from build123d import *

# Parameters (mm, degrees)
F1_DEPTH = 50
F4_DEPTH = 31
F5_R     = 26
F6_DEPTH = 15


with BuildPart() as f1:
    # F0 (on Front) → F1 (new body)
    with BuildSketch(Plane.XZ):
        with BuildLine():
            ThreePointArc((55.5, 51.9206124771), (30.2492433933, 69.7207521053), (0, 76))
            ThreePointArc((0, 76), (-76, 0), (0, -76))
            ThreePointArc((0, -76), (30.2492433933, -69.7207521053), (55.5, -51.9206124771))
            ThreePointArc((55.5, -51.9206124771), (35, 0), (55.5, 51.9206124771))
        make_face()
        with BuildLine():
            ThreePointArc((111, 76), (80.7507566067, 69.7207521053), (55.5, 51.9206124771))
            ThreePointArc((55.5, 51.9206124771), (70.6894617323, 27.9105714739), (76, 0))
            ThreePointArc((76, 0), (70.6894617323, -27.9105714739), (55.5, -51.9206124771))
            ThreePointArc((55.5, -51.9206124771), (80.7507566067, -69.7207521053), (111, -76))
            ThreePointArc((111, -76), (164.7401153702, -53.7401153702), (187, 0))
            ThreePointArc((187, 0), (164.7401153702, 53.7401153702), (111, 76))
        make_face()
        with BuildLine():
            ThreePointArc((76, 0), (70.6894617323, 27.9105714739), (55.5, 51.9206124771))
            ThreePointArc((55.5, 51.9206124771), (35, 0), (55.5, -51.9206124771))
            ThreePointArc((55.5, -51.9206124771), (70.6894617323, -27.9105714739), (76, 0))
        make_face()
        with BuildLine():
            Line((111, 76), (0, 76))
            ThreePointArc((0, 76), (30.2492433933, 69.7207521053), (55.5, 51.9206124771))
            ThreePointArc((55.5, 51.9206124771), (80.7507566067, 69.7207521053), (111, 76))
        make_face()
        with BuildLine():
            ThreePointArc((55.5, -51.9206124771), (30.2492433933, -69.7207521053), (0, -76))
            Line((0, -76), (111, -76))
            ThreePointArc((111, -76), (80.7507566067, -69.7207521053), (55.5, -51.9206124771))
        make_face()
    extrude(amount=F1_DEPTH)

    # F3 (on offset) → F4 (cut)
    with BuildSketch(Plane.XZ.offset(19)):
        with BuildLine():
            Line((111, 64), (0, 64))
            ThreePointArc((0, 64), (-64, 0), (0, -64))
            Line((0, -64), (111, -64))
            ThreePointArc((111, -64), (175, 0), (111, 64))
        make_face()
    extrude(amount=F4_DEPTH, mode=Mode.SUBTRACT)

    # F5 (on face) → F6 (cut)
    with BuildSketch(Plane.XZ.offset(19)):
        Circle(F5_R)
    extrude(amount=-F6_DEPTH, mode=Mode.SUBTRACT)

    # F8 (on offset) → F9 (revolve, cut)
    with BuildSketch(Plane.YZ.offset(111)):
        Polygon((-19, 0), (0, 0), (0, 11), (-2, 11), (-2, 18.5), (-7, 18.5), (-7, 23.5), (-19, 23.5), align=None)
    revolve(axis=Axis((111, -31.2652774155, 0), (0, -1, 0)), mode=Mode.SUBTRACT)


solid = f1.part
For this review, take the finished solid that the model builds, in its own axes (mm). A direction names the side the tool comes from. Coordinates: 2 decimals unless noted, no trailing zeros. Loops run counter-clockwise (first coordinate to the right, second up) from the corner with the lowest first, then second, coordinate; pieces in that order, holes last. Notation, with made-up numbers: (-7.5, 80) -> (30.5, 80) arc R19 cw to (30.5, 89) -> close; hole circle Ø5 at (16, 56.5). An arc over 180 degrees is marked (long way). Write each question's results on one line, items separated by ' | '.
Q1. To check wall thickness, follow line 1 along Z through (x, y) = (5, -46.5); line 2 along X through (y, z) = (-40.5, -2.5); line 3 along X through (y, z) = (-8, 3). State the ranges of each line that lie inside material, in increasing order. Write a range as [from, to].
Taken from the geometry:
line 1: [-76, -64], [64, 76] | line 2: [-75.96, -63.95], [174.95, 186.96] | line 3: [-75.94, -25.83], [25.83, 87.69], [134.31, 186.94]
Q2. Add section B-B, the plane x = 46.5. State the section outline as (y, z) points, then the cut area to 3 significant figures.
Taken from the geometry:
outline: (-50, -76) -> (0, -76) -> (0, 76) -> (-50, 76) -> (-50, 64) -> (-19, 64) -> (-19, -64) -> (-50, -64) -> close | area: 3,630 mm²
Q3. Mouldability with a two-part tool opening along Z and no side actions: class faces 1 (the cylindrical face through (-75.98, -24.65, 1.67)), 2 (the cylindrical face through (129.06, -4.54, -4.01)), 3 (the flat face through (55, -50, -67)), 4 (the flat face through (56, -25, 76)) as +Z half, -Z half, draft (parallel to the pull), parting line (faces both ways), or undercut.
Taken from the geometry:
face 1: parting line | face 2: undercut | face 3: draft | face 4: +Z half
Q4. Machinability: for faces 5 (the flat face through (0, -4, 0)), 6 (the flat face through (55, -25, -76)), which of the approach directions +Z, -Z, +X, -X, +Y, -Y give a long, thin tool a straight path to every point of the face, cutting with its end or side? Answer none if there is none.
Taken from the geometry:
face 5: -Y | face 6: -Z, +X, -X, +Y, -Y
Q5. For pin 1 Ø18.5 at (x, z) = (108, 0.5) entering from -Y; pin 2 Ø12 at (y, z) = (-39, -9.5) entering from +X; pin 3 Ø2 at (y, z) = (-7, -45.5) entering from +X, all flat-tipped, find the tip position at first contact; note any pin that passes through.
Taken from the geometry:
pin 1: y = -2 | pin 2: x = 186.92 | pin 3: x = 172.61
Q6. Add section D-D, the plane x = -30.5. State the section outline as (y, z) points (3 decimals), then the cut area to 3 significant figures.
Taken from the geometry:
outline: (-50, -69.611) -> (0, -69.611) -> (0, 69.611) -> (-50, 69.611) -> (-50, 56.265) -> (-19, 56.265) -> (-19, -56.265) -> (-50, -56.265) -> close | area: 3,470 mm²
Q7. Add section A-A, the plane y = -44.5. State the section outline as (x, z) points, then the cut area to 3 significant figures.
Taken from the geometry:
outline: (0, -76) -> (111, -76) arc R76 ccw to (111, 76) -> (0, 76) arc R76 ccw to start; hole (0, -64) -> (111, -64) arc R64 ccw to (111, 64) -> (0, 64) arc R64 ccw to start | area: 7,940 mm²
Q8. Add section C-C, the plane z = -6. State the section outline as (x, y) points, then the cut area to 3 significant figures.
Taken from the geometry:
outline: (-75.76, -50) -> (-63.72, -50) -> (-63.72, -19) -> (-25.3, -19) -> (-25.3, -4) -> (25.3, -4) -> (25.3, -19) -> (88.28, -19) -> (88.28, -7) -> (93.5, -7) -> (93.5, -2) -> (101.78, -2) -> (101.78, 0) -> (-75.76, 0) -> close; (120.22, -2) -> (128.5, -2) -> (128.5, -7) -> (133.72, -7) -> (133.72, -19) -> (174.72, -19) -> (174.72, -50) -> (186.76, -50) -> (186.76, 0) -> (120.22, 0) -> close | area: 4,220 mm²
